```python
from build123d import *

# Parameters (mm, degrees)
SKETCH_1_W                   = 48
SKETCH_1_H                   = 55
EXTRUDE_1_DEPTH              = 5.5
HOLE_WIZARD_M5_1_D           = 5.5
HOLE_WIZARD_M5_1_CBORE_D     = 10
HOLE_WIZARD_M5_1_CBORE_DEPTH = 5.4
MIRROR_2_COPY_1_D            = 5.5
MIRROR_2_COPY_1_CBORE_D      = 10
MIRROR_2_COPY_1_CBORE_DEPTH  = 5.4
SKETCH_4_W                   = 48
SKETCH_4_H                   = 11
EXTRUDE_2_DEPTH              = 64.277224085
SKETCH_5_R                   = 2.5
CUT_EXTRUDE_1_DEPTH          = 96.498999266


with BuildPart() as part:
    # 草图1 → 凸台-拉伸1 (new, symmetric)
    with BuildSketch(Plane.XY):
        Rectangle(SKETCH_1_W, SKETCH_1_H)
    extrude(amount=EXTRUDE_1_DEPTH, both=True)

    # M5 六角凹头螺钉的柱形沉头孔1 (through all)
    with Locations(Plane(origin=(-7.5, -20, 5.5), x_dir=(1, 0, 0), z_dir=(0, 0, 1))):
        with Locations((0, 0)):
            hole_wizard_m5_1 = CounterBoreHole(HOLE_WIZARD_M5_1_D / 2, HOLE_WIZARD_M5_1_CBORE_D / 2, HOLE_WIZARD_M5_1_CBORE_DEPTH)

    # 镜向1: M5 六角凹头螺钉的柱形沉头孔1 across plane
    add(hole_wizard_m5_1.mirror(Plane(origin=(0, 0, 0), x_dir=(0, 0, 1), z_dir=(1, 0, 0))), mode=Mode.SUBTRACT)

    # 镜向2: M5 六角凹头螺钉的柱形沉头孔1 across plane
    add(hole_wizard_m5_1.mirror(Plane.ZX), mode=Mode.SUBTRACT)

    # 镜向2 copy 1 (through all)
    with Locations(Plane(origin=(7.5, 20, 5.5), x_dir=(-1, 0, 0), z_dir=(0, 0, 1))):
        with Locations((0, 0)):
            CounterBoreHole(MIRROR_2_COPY_1_D / 2, MIRROR_2_COPY_1_CBORE_D / 2, MIRROR_2_COPY_1_CBORE_DEPTH)

    # 草图4 → 凸台-拉伸2 (add)
    with BuildSketch(Plane.XZ.offset(27.5)):
        Rectangle(SKETCH_4_W, SKETCH_4_H)
    extrude(amount=EXTRUDE_2_DEPTH)

    # 草图5 → 切除-拉伸1 (cut, through all)
    with BuildSketch(Plane.XY.offset(5.5)):
        with Locations((-9.3, -81.777224085)):
            Circle(SKETCH_5_R)
        with Locations((9.3, -81.777224085)):
            Circle(SKETCH_5_R)
    extrude(amount=-CUT_EXTRUDE_1_DEPTH, mode=Mode.SUBTRACT)


solid = part.part
```
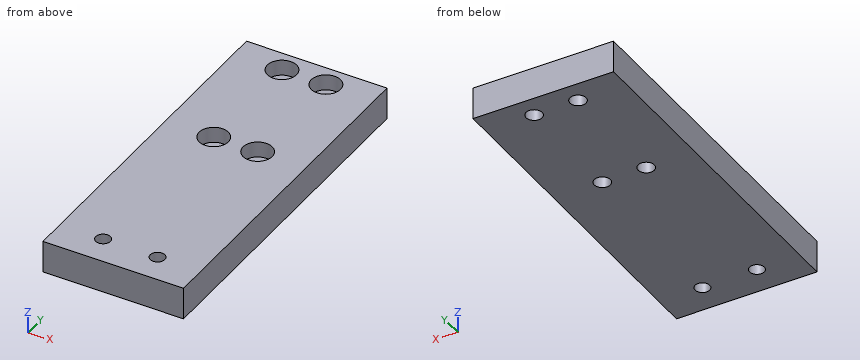
The listing builds one solid part. Answer for the finished solid, in the listing's coordinates (mm). Round coordinates to 2 decimals unless told otherwise and drop trailing zeros. Order: outer loops, then holes, each group sorted by start corner. A loop starts at its lowest first (then second) coordinate and runs counter-clockwise, first axis right, second up. Notation, with made-up numbers: (-5, -22.75) -> (31, -22.75) arc R11 cw to (31, -1.75) -> close; hole circle Ø7 at (42, 16.5). An arc over 180 degrees is marked (long way). Answer as CSV lines item,"result".
Q1. Consider line 1 (X direction, y = 20, z = -3.35); line 2 (X direction, y = -18, z = -1.5); line 3 (Y direction, x = -7.5, z = 2.25). Determine where each line is inside the solid, lowest interval first. Write a range as from..to.
Computed values:
line 1,"x = -24..-10.25, -4.75..4.75, 10.25..24"
line 2,"x = -24..-9.39, -5.61..5.61, 9.39..24"
line 3,"y = -91.78..-83.51, -80.04..-25, -15..15, 25..27.5"
Q2. Given pin 1 (5 mm diameter, centred on x = 6, y = -20, fed in from +Z); pin 2 (5 mm diameter, centred on x = -7.5, y = 20, fed in from +Z), each flat-ended and moving along its own axis, determine where each tip first touches the part or whether it passes through.
Computed values:
pin 1,"stops at z = 0.1"
pin 2,"passes through"
Q3. A cutting plane is placed at A-A on y = -20. Determine the outline of the cut face in (x, z), plus the area to 3 significant figures.
Computed values:
outline,"(-24, -5.5) -> (-10.25, -5.5) -> (-10.25, 0.1) -> (-12.5, 0.1) -> (-12.5, 5.5) -> (-24, 5.5) -> close; (-4.75, -5.5) -> (4.75, -5.5) -> (4.75, 0.1) -> (2.5, 0.1) -> (2.5, 5.5) -> (-2.5, 5.5) -> (-2.5, 0.1) -> (-4.75, 0.1) -> close; (10.25, -5.5) -> (24, -5.5) -> (24, 5.5) -> (12.5, 5.5) -> (12.5, 0.1) -> (10.25, 0.1) -> close"
area,"358 mm^2"
Q4. A cutting plane is placed at B-B on z = -3.25. Determine the outline of the cut face in (x, y).
Computed values:
outline,"(-24, -91.78) -> (24, -91.78) -> (24, 27.5) -> (-24, 27.5) -> close; hole circle Ø5 at (-9.3, -81.78); hole circle Ø5.5 at (-7.5, -20); hole circle Ø5.5 at (-7.5, 20); hole circle Ø5.5 at (7.5, -20); hole circle Ø5.5 at (7.5, 20); hole circle Ø5 at (9.3, -81.78)"
